Build history of the part. All positions in model axes, mm. A direction names the side the tool comes from. Give positions to 0.01 mm unless a question says otherwise; leave off trailing zeros. Order: outer loops, then holes, each group sorted by start corner. A loop starts at its lowest first (then second) coordinate and runs counter-clockwise, first axis right, second up. Notation, with made-up numbers: (79, 67) - (109, 67) arc R32 ccw to (109, 100) - close; hole circle Ø3 at (-38, 52). An arc over 180 degrees is marked (long way). Use a Markdown table: item, result. Add a question column.
(1) Mould opens along X. For faces 5 (the face through (0, 1, -4)), 6 (the face through (-13.88, 0.94, -3.47)), 7 (the face through (-6.375, 0.939, -3.093)), 8 (the face through (16.47, 0.94, 0.03)) say: +X half, -X half, draft (parallel to the pull), parting line (faces both ways), or undercut.
(2) Which spindle directions (+Z, -Z, +X, -X, +Y, -Y) get a long thin tool onto all of the face, cutting with end or side? Do faces 1 (the face through (-10.41, 0.94, 3.94)), 2 (the face through (8.8, 2.4, -3.4)), 3 (the face through (0, 1, 4)), 4 (the face through (8.75, 0.94, -3.63)). Say none if no direction does.
(3) Slice it at B-B (z = 0). Count the separate pieces of the cut face and the enclosed holes in it, then the cut area to 3 significant figures.
(4) Flat gauge pins, fed straight in: pin 1 (0.6 mm diameter, centred on x = 0, y = 1, fed in from -Z); pin 2 (1.5 mm diameter, centred on x = -0.5, y = 1, fed in from +Z). Where does each tip first touch, or does it go through?
(5) Wall check: line 1 (Z direction, x = 0, y = 0.6) (3 decimals); line 2 (X direction, y = 2.45, z = 1.25); line 3 (X direction, y = 2.2, z = 0.5). Give the ranges that are in metal, low to high.
(6) Slice it at A-A (x = 0). Write the cut outline in (y, z) (3 decimals).
from build123d import *

# Parameters (mm, degrees)
BOSS_EXTRUDE3_DEPTH = 2.54
FILLET1_R           = 6.35
FILLET2_R           = 0.635


with BuildPart() as part:
    # Sketch2 → Boss-Extrude3 (new body)
    with BuildSketch(Plane(origin=(0, 0, 0), x_dir=(1, 0, 0), z_dir=(0, 1, 0))):
        with BuildLine():
            ThreePointArc((-14.9225, 0), (-12.7, 2.2225), (-10.4775, 0))
            Line((-10.4775, 0), (-8.081142289, 0))
            Line((-8.081142289, 0), (-9.450372471, 2.371576242))
            Line((-9.450372471, 2.371576242), (-10.390571145, 4.000048114))
            Line((-10.390571145, 4.000048114), (-15.009428855, 4.000048114))
            Line((-15.009428855, 4.000048114), (-17.318857711, 0))
            Line((-17.318857711, 0), (-14.9225, 0))
        make_face()
        with BuildLine():
            Line((-8.081142289, 0), (-10.4775, 0))
            ThreePointArc((-10.4775, 0), (-12.7, -2.2225), (-14.9225, 0))
            Line((-14.9225, 0), (-17.318857711, 0))
            Line((-17.318857711, 0), (-15.009428855, -4.000048114))
            Line((-15.009428855, -4.000048114), (-10.390571145, -4.000048114))
            Line((-10.390571145, -4.000048114), (-9.235856717, -2.000024057))
            Line((-9.235856717, -2.000024057), (-8.081142289, 0))
        make_face()
        Polygon((-9.450372471, 2.371576242), (-8.081142289, 0), (-4.618857711, 0), (-3.464143283, 2.000024057), (-2.309428855, 4.000048114), (-6.35, 2.833322689), (-10.390571145, 4.000048114), align=None)
        Polygon((-4.618857711, 0), (-8.081142289, 0), (-9.235856717, -2.000024057), (-10.390571145, -4.000048114), (-6.35, -2.833322689), (-2.309428855, -4.000048114), (-3.464143283, -2.000024057), align=None)
        with BuildLine():
            Line((-3.464143283, 2.000024057), (-4.618857711, 0))
            Line((-4.618857711, 0), (-2.025, 0))
            ThreePointArc((-2.025, 0), (0, 2.025), (2.025, 0))
            Line((2.025, 0), (4.618857711, 0))
            Line((4.618857711, 0), (3.464143283, 2.000024057))
            Line((3.464143283, 2.000024057), (2.309428855, 4.000048114))
            Line((2.309428855, 4.000048114), (-2.309428855, 4.000048114))
            Line((-2.309428855, 4.000048114), (-3.464143283, 2.000024057))
        make_face()
        with BuildLine():
            Line((-2.025, 0), (-4.618857711, 0))
            Line((-4.618857711, 0), (-3.464143283, -2.000024057))
            Line((-3.464143283, -2.000024057), (-2.309428855, -4.000048114))
            Line((-2.309428855, -4.000048114), (2.309428855, -4.000048114))
            Line((2.309428855, -4.000048114), (3.464143283, -2.000024057))
            Line((3.464143283, -2.000024057), (4.618857711, 0))
            Line((4.618857711, 0), (2.025, 0))
            ThreePointArc((2.025, 0), (0, -2.025), (-2.025, 0))
        make_face()
        Polygon((3.464143283, 2.000024057), (4.618857711, 0), (7.946932116, 0), (9.135199087, 2.058138767), (10.323466058, 4.116277534), (6.282791089, 2.86963953), (2.309428855, 4.000048114), align=None)
        Polygon((7.946932116, 0), (4.618857711, 0), (3.464143283, -2.000024057), (2.309428855, -4.000048114), (6.282791089, -2.86963953), (10.323466058, -4.116277534), (9.135199087, -2.058138767), align=None)
        with BuildLine():
            Line((9.135199087, 2.058138767), (7.946932116, 0))
            Line((7.946932116, 0), (10.4775, 0))
            ThreePointArc((10.4775, 0), (12.7, 2.2225), (14.9225, 0))
            Line((14.9225, 0), (17.453067884, 0))
            Line((17.453067884, 0), (15.076533942, 4.116277534))
            Line((15.076533942, 4.116277534), (10.323466058, 4.116277534))
            Line((10.323466058, 4.116277534), (9.135199087, 2.058138767))
        make_face()
        with BuildLine():
            Line((10.4775, 0), (7.946932116, 0))
            Line((7.946932116, 0), (9.135199087, -2.058138767))
            Line((9.135199087, -2.058138767), (10.323466058, -4.116277534))
            Line((10.323466058, -4.116277534), (15.076533942, -4.116277534))
            Line((15.076533942, -4.116277534), (17.453067884, 0))
            Line((17.453067884, 0), (14.9225, 0))
            ThreePointArc((14.9225, 0), (12.7, -2.2225), (10.4775, 0))
        make_face()
    extrude(amount=BOSS_EXTRUDE3_DEPTH)

    # Fillet1
    # the kernel refuses this fillet: 6.35 mm, written as the material it adds along each edge
    with BuildSketch(Plane(origin=(-6.35, 0, -2.833322689), x_dir=(-0.9607490883142406, 0, -0.2774187976748433), z_dir=(0, 1, 0)), Plane(origin=(-6.35, 0, 2.833322689), x_dir=(0.9607490883142819, 0, 0.27741879767470035), z_dir=(0, 1, 0))) as fillet1_piece_1:
        with BuildLine():
            CenterArc((FILLET1_R * 0.288752600496, -FILLET1_R), FILLET1_R, 90, 32.212421432)
            Line((-FILLET1_R * 0.244307113399, -FILLET1_R * 0.153922378607), (0, 0))
            Line((0, 0), (FILLET1_R * 0.288752600496, 0))
        make_face()
    extrude(amount=2.54)
    with BuildSketch(Plane(origin=(6.282791089, 0, -2.86963953), x_dir=(-0.9618326798752038, 0, -0.27363825742041953), z_dir=(0, 1, 0)), Plane(origin=(6.282791089, 0, 2.86963953), x_dir=(0.9555558296704232, 0, 0.2948102040005893), z_dir=(0, 1, 0))) as fillet1_piece_2:
        with BuildLine():
            CenterArc((FILLET1_R * 0.296470151245, -FILLET1_R), FILLET1_R, 90, 33.027036352)
            Line((-FILLET1_R * 0.248564569422, -FILLET1_R * 0.16158652607), (0, 0))
            Line((0, 0), (FILLET1_R * 0.296470151245, 0))
        make_face()
    extrude(amount=2.54)
    # the kernel refuses this fillet: 6.35 mm, written as the material it takes off along each edge
    with BuildSketch(Plane(origin=(-10.390571145, -2.246092292, -4.000048114), x_dir=(-1, 0, 0), z_dir=(0, 1, 0))) as fillet1_2_piece_1:
        with BuildLine():
            CenterArc((FILLET1_R * 0.141486128607, FILLET1_R), FILLET1_R, 253.893789284, 16.106210716)
            Line((-FILLET1_R * 0.135932669068, FILLET1_R * 0.0392509116858), (0, 0))
            Line((0, 0), (FILLET1_R * 0.141486128607, 0))
        make_face()
    extrude(amount=7.032184583, mode=Mode.SUBTRACT)
    with BuildSketch(Plane(origin=(-2.309428855, -2.246092292, -4.000048114), x_dir=(1, 0, 0), z_dir=(0, 1, 0)), Plane(origin=(-2.309428855, -2.246092292, 4.000048114), x_dir=(-0.9607490883142817, 0, -0.2774187976747005), z_dir=(0, 1, 0)), Plane(origin=(-10.390571145, -2.246092292, 4.000048114), x_dir=(-1, 0, 0), z_dir=(0, 1, 0))) as fillet1_2_piece_2:
        with BuildLine():
            CenterArc((FILLET1_R * 0.141486128607, -FILLET1_R), FILLET1_R, 90, 16.106210716)
            Line((-FILLET1_R * 0.135932669068, -FILLET1_R * 0.0392509116857), (0, 0))
            Line((0, 0), (FILLET1_R * 0.141486128607, 0))
        make_face()
    extrude(amount=7.032184583, mode=Mode.SUBTRACT)
    with BuildSketch(Plane(origin=(2.309428855, -2.214259851, -4.000048114), x_dir=(0.9618326798752038, 0, 0.27363825742041936), z_dir=(0, 1, 0)), Plane(origin=(2.309428855, -2.214259851, 4.000048114), x_dir=(-1, 0, 0), z_dir=(0, 1, 0))) as fillet1_2_piece_3:
        with BuildLine():
            CenterArc((FILLET1_R * 0.139480935468, -FILLET1_R), FILLET1_R, 90, 15.880879627)
            Line((-FILLET1_R * 0.134157321953, -FILLET1_R * 0.0381673201248), (0, 0))
            Line((0, 0), (FILLET1_R * 0.139480935468, 0))
        make_face()
    extrude(amount=6.968519701, mode=Mode.SUBTRACT)
    with BuildSketch(Plane(origin=(10.323466058, -2.39323875, -4.116277534), x_dir=(1, 0, 0), z_dir=(0, 1, 0)), Plane(origin=(10.323466058, -2.39323875, 4.116277534), x_dir=(-0.9555558296704234, 0, -0.294810204000589), z_dir=(0, 1, 0))) as fillet1_2_piece_4:
        with BuildLine():
            CenterArc((FILLET1_R * 0.150755196823, -FILLET1_R), FILLET1_R, 90, 17.146156725)
            Line((-FILLET1_R * 0.144055007178, -FILLET1_R * 0.0444441703296), (0, 0))
            Line((0, 0), (FILLET1_R * 0.150755196823, 0))
        make_face()
    extrude(amount=7.326477499, mode=Mode.SUBTRACT)
    with BuildSketch(Plane(origin=(15.076533942, -9.165435523, -4.116277534), x_dir=(0.500000000000005, 0, 0.8660254037844358), z_dir=(0, 1, 0)), Plane(origin=(17.453067884, -9.165435523, 0), x_dir=(-0.49999999999999534, 0, 0.8660254037844413), z_dir=(0, 1, 0)), Plane(origin=(15.076533942, -9.165435523, 4.116277534), x_dir=(-1, 0, 0), z_dir=(0, 1, 0)), Plane(origin=(-15.009428855, -9.165435523, 4.000048114), x_dir=(-0.5000000000000033, 0, -0.8660254037844367), z_dir=(0, 1, 0)), Plane(origin=(-17.318857711, -9.165435523, 0), x_dir=(0.4999999999999972, 0, -0.8660254037844403), z_dir=(0, 1, 0)), Plane(origin=(-15.009428855, -9.165435523, -4.000048114), x_dir=(1, 0, 0), z_dir=(0, 1, 0))) as fillet1_2_piece_5:
        with BuildLine():
            CenterArc((FILLET1_R * 0.57735026919, -FILLET1_R), FILLET1_R, 90, 60)
            Line((-FILLET1_R * 0.288675134595, -FILLET1_R * 0.5), (0, 0))
            Line((0, 0), (FILLET1_R * 0.57735026919, 0))
        make_face()
    extrude(amount=20.870871047, mode=Mode.SUBTRACT)

    # Fillet2
    fillet2_edges = [part.edges().sort_by_distance(p)[0] for p in [
        (-2.025, 2.54, 0),
        (-8.819504031, 2.54, -3.546398399),
        (8.745211682, 2.54, 3.629350993),
        (11.345560645, 2.54, 4.116277534),
        (11.345560645, 2.54, -4.116277534),
        (8.745211682, 2.54, -3.629350993),
        (3.81669336, 2.54, -3.571236283),
        (0.006366488, 2.54, -4.000048114),
        (-3.880495969, 2.54, -3.546398399),
        (-11.316131354, 2.54, 4.000048114),
        (-8.819504031, 2.54, 3.546398399),
        (-3.880495969, 2.54, 3.546398399),
        (0.006366488, 2.54, 4.000048114),
        (3.81669336, 2.54, 3.571236283),
        (-13.908962899, 2.54, -3.458631518),
        (-16.336509292, 2.54, 0),
        (-13.908962899, 2.54, 3.458631518),
        (-10.399430946, 2.54, 3.937428535),
        (-2.300569054, 2.54, 3.937428535),
        (2.30093691, 2.54, 3.939165629),
        (10.334162366, 2.54, 4.045326026),
        (14.007411183, 2.54, 3.560915034),
        (16.470719465, 2.54, 0),
        (14.007411183, 2.54, -3.560915034),
        (10.334162366, 2.54, -4.045326026),
        (2.30093691, 2.54, -3.939165629),
        (-2.300569054, 2.54, -3.937428535),
        (-10.399430946, 2.54, -3.937428535),
        (-6.35, 2.54, -3.092748685),
        (6.279774704, 2.54, -3.142811536),
        (6.279774704, 2.54, 3.142811536),
        (-6.35, 2.54, 3.092748685),
        (-11.316131354, 2.54, -4.000048114),
    ]]
    fillet(fillet2_edges, radius=FILLET2_R)


solid = part.part
Solution:
| question | item | result |
|---|---|---|
| 1 | face 5 | draft |
| 1 | face 6 | -X half |
| 1 | face 7 | undercut |
| 1 | face 8 | +X half |
| 2 | face 1 | +Z, +Y, -Y |
| 2 | face 2 | -Z, +Y |
| 2 | face 3 | +Z, -X, +Y, -Y |
| 2 | face 4 | -Z, +Y, -Y |
| 3 | separate pieces | 4 |
| 3 | enclosed holes | 0 |
| 3 | area | 50.1 mm2 |
| 4 | pin 1 | z = -4 |
| 4 | pin 2 | z = 4 |
| 5 | line 1 | -4 to -2.025, 2.025 to 4 |
| 5 | line 2 | -15.9 to -14.54, -10.86 to -1.97, 1.97 to 10.86, 14.54 to 16.03 |
| 5 | line 3 | -16.24 to -14.87, -10.53 to -2.04, 2.04 to 10.53, 14.87 to 16.38 |
| 6 | outline | (0, -4) - (1.905, -4) arc R0.635 ccw to (2.54, -3.365) - (2.54, -2.66) arc R0.635 ccw to (1.905, -2.025) - (0, -2.025) - close; (0, 2.025) - (1.905, 2.025) arc R0.635 ccw to (2.54, 2.66) - (2.54, 3.365) arc R0.635 ccw to (1.905, 4) - (0, 4) - close |
